from build123d import *

# Parameters (mm, degrees)
F0_W        = 100
F0_H        = 100
F1_DEPTH    = 50
F2_R        = 10
F3_T1_DEPTH = 150
F3_T4_ANGLE = 90
F3_T6_ANGLE = 90
F4_T1_DEPTH = 87.5
F4_T4_ANGLE = 90
F4_T6_ANGLE = 90
F5_R        = 30.8330010445
F6_DEPTH    = 40


# Not quite as in the source:
# - a fillet or chamfer that OpenCascade refuses, or shapes differently, is made with other operations: its cross-section is extruded or revolved along the edge and cut away or added


with BuildPart() as f1:
    # F0 (on Top) → F1 (new body)
    with BuildSketch(Plane.XY):
        with Locations((-16.9892802835, -14.8166164756)):
            Rectangle(F0_W, F0_H)
    extrude(amount=F1_DEPTH)

    # F2
    f2_edges = [f1.edges().sort_by_distance(p)[0] for p in [
        (-16.98928, -64.816616, 50),
        (33.01072, -14.816616, 50),
        (-16.98928, 35.183384, 50),
        (-66.98928, -14.816616, 50),
    ]]
    fillet(f2_edges, radius=F2_R)

    # F3: fillet of radius 40 on 2 edges, made by hand

    # F3_s2 → F3_t1 (cut)
    with BuildSketch(Plane.XY.offset(-100)):
        with BuildLine():
            ThreePointArc((33.0107197165, -24.8166164756), (21.294990964, -53.100887723), (-6.9892802835, -64.8166164756))
            Line((-6.9892802835, -64.8166164756), (33.0107197165, -64.8166164756))
            Line((33.0107197165, -64.8166164756), (33.0107197165, -24.8166164756))
        make_face()
        with BuildLine():
            ThreePointArc((-26.9892802835, 35.1833835244), (-55.2735515309, 23.4676547719), (-66.9892802835, -4.8166164756))
            Line((-66.9892802835, -4.8166164756), (-66.9892802835, 35.1833835244))
            Line((-66.9892802835, 35.1833835244), (-26.9892802835, 35.1833835244))
        make_face()
    extrude(amount=F3_T1_DEPTH, mode=Mode.SUBTRACT)

    # F3_s3 → F3_t4 (revolve, cut)
    with BuildSketch(Plane.YZ.offset(-26.9892802835)):
        with BuildLine():
            ThreePointArc((25.1833835244, 50), (32.2544513363, 47.0710678119), (35.1833835244, 40))
            Line((35.1833835244, 40), (35.1833835244, 50))
            Line((35.1833835244, 50), (25.1833835244, 50))
        make_face()
    revolve(axis=Axis((-26.9892802835, -4.8166164756, 50), (0, 0, 1)), revolution_arc=F3_T4_ANGLE, mode=Mode.SUBTRACT)

    # F3_s5 → F3_t6 (revolve, cut)
    with BuildSketch(Plane.YZ.offset(-6.9892802835)):
        with BuildLine():
            ThreePointArc((-54.8166164756, 50), (-61.8876842874, 47.0710678119), (-64.8166164756, 40))
            Line((-64.8166164756, 40), (-64.8166164756, 50))
            Line((-64.8166164756, 50), (-54.8166164756, 50))
        make_face()
    revolve(axis=Axis((-6.9892802835, -24.8166164756, 50), (0, 0, 1)), revolution_arc=F3_T6_ANGLE, mode=Mode.SUBTRACT)

    # F4: fillet of radius 15 on 2 edges, made by hand

    # F4_s2 → F4_t1 (cut)
    with BuildSketch(Plane.XY.offset(-37.5)):
        with BuildLine():
            ThreePointArc((33.0107197165, 20.1833835244), (28.6173214343, 30.7899852422), (18.0107197165, 35.1833835244))
            Line((18.0107197165, 35.1833835244), (33.0107197165, 35.1833835244))
            Line((33.0107197165, 35.1833835244), (33.0107197165, 20.1833835244))
        make_face()
        with BuildLine():
            ThreePointArc((-51.9892802835, -64.8166164756), (-62.5958820012, -60.4232181934), (-66.9892802835, -49.8166164756))
            Line((-66.9892802835, -49.8166164756), (-66.9892802835, -64.8166164756))
            Line((-66.9892802835, -64.8166164756), (-51.9892802835, -64.8166164756))
        make_face()
    extrude(amount=F4_T1_DEPTH, mode=Mode.SUBTRACT)

    # F4_s3 → F4_t4 (revolve, cut)
    with BuildSketch(Plane.XZ.offset(49.8166164756)):
        with BuildLine():
            ThreePointArc((-56.9892802835, 50), (-64.0603480953, 47.0710678119), (-66.9892802835, 40))
            Line((-66.9892802835, 40), (-66.9892802835, 50))
            Line((-66.9892802835, 50), (-56.9892802835, 50))
        make_face()
    revolve(axis=Axis((-51.9892802835, -49.8166164756, 50), (0, 0, 1)), revolution_arc=F4_T4_ANGLE, mode=Mode.SUBTRACT)

    # F4_s5 → F4_t6 (revolve, cut)
    with BuildSketch(Plane.XZ.offset(-20.1833835244)):
        with BuildLine():
            ThreePointArc((23.0107197165, 50), (30.0817875284, 47.0710678119), (33.0107197165, 40))
            Line((33.0107197165, 40), (33.0107197165, 50))
            Line((33.0107197165, 50), (23.0107197165, 50))
        make_face()
    revolve(axis=Axis((18.0107197165, 20.1833835244, 50), (0, 0, 1)), revolution_arc=F4_T6_ANGLE, mode=Mode.SUBTRACT)

    # F5 (on face) → F6 (cut)
    with BuildSketch(Plane.XY.offset(50)):
        with Locations((-16.8512575328, -14.6785899997)):
            Circle(F5_R)
    extrude(amount=-F6_DEPTH, mode=Mode.SUBTRACT)


solid = f1.part
Verification items for the finished model (mm, model axes). Round coordinates to 2 decimals unless told otherwise and drop trailing zeros. Loops run counter-clockwise (first coordinate to the right, second up) from the corner with the lowest first, then second, coordinate; pieces in that order, holes last. Notation, with made-up numbers: (-25, -40) - (-13, -40) arc R23 cw to (-13, -7) - close; hole circle Ø10 at (30, 53). An arc over 180 degrees is marked (long way). Answer in a Markdown table with one row per item. Add a question column.
Q1. Section check A-A on z = 25. Enter the section's corners in (x, y), plus the area to 3 significant figures.
Q2. Section check C-C on y = -21.5. Enter the section's corners in (x, z).
Q3. Section check B-B on z = 5. Enter the section's corners in (x, y).
Q4. Release check for a two-part mould opening along X. For faces 1 (the face through (-17, -14, 10)), 2 (the face through (-29.17, -61.97, 46.99)), 3 (the face through (12.56, -5.42, 30.28)), 4 (the face through (30.16, -2, 46.99)) record: pulls with the +X half, pulls with the -X half, needs draft (parallel to the pull), parting line crosses it, or undercut.
Q5. Gauge pin test, flat ends, axial feed: pin 1 (18.5 mm diameter, centred on x = -23.5, y = -30, fed in from +Z); pin 2 (1 mm diameter, centred on x = -28.5, z = 12, fed in from +Y); pin 3 (8 mm diameter, centred on y = -37, z = 11.5, fed in from +X). Record the tip position at first contact, or that the pin passes through.
Q6. Material ranges on line 1 (Z direction, x = 7, y = -26.5); line 2 (X direction, y = 6.5, z = 33.5); line 3 (X direction, y = 12.5, z = 38.5), recorded low to high.
Q7. Section check D-D on x = -15.5. Enter the section's corners in (y, z).
Found:
| question | item | result |
|---|---|---|
| 1 | outline | (-66.99, -49.82) arc R15 ccw to (-51.99, -64.82) - (-6.99, -64.82) arc R40 ccw to (33.01, -24.82) - (33.01, 20.18) arc R15 ccw to (18.01, 35.18) - (-26.99, 35.18) arc R40 ccw to (-66.99, -4.82) - close; hole circle Ø61.67 at (-16.85, -14.68) |
| 1 | area | 6,230 mm² |
| 2 | outline | (-66.99, 0) - (33.01, 0) - (33.01, 40) arc R10 ccw to (23.01, 50) - (13.22, 50) - (13.22, 10) - (-46.92, 10) - (-46.92, 50) - (-56.99, 50) arc R10 ccw to (-66.99, 40) - close |
| 3 | outline | (-66.99, -49.82) arc R15 ccw to (-51.99, -64.82) - (-6.99, -64.82) arc R40 ccw to (33.01, -24.82) - (33.01, 20.18) arc R15 ccw to (18.01, 35.18) - (-26.99, 35.18) arc R40 ccw to (-66.99, -4.82) - close |
| 4 | face 1 | undercut |
| 4 | face 2 | needs draft |
| 4 | face 3 | undercut |
| 4 | face 4 | pulls with the +X half |
| 5 | pin 1 | stops at z = 10 |
| 5 | pin 2 | stops at y = 35.17 |
| 5 | pin 3 | stops at x = 32.16 |
| 6 | line 1 | z = 0 to 10 |
| 6 | line 2 | x = -65.36 to -39.26, 5.56 to 33.01 |
| 6 | line 3 | x = -63.05 to -31.41, -2.29 to 33.01 |
| 7 | outline | (-64.82, 0) - (35.18, 0) - (35.18, 40) arc R10 ccw to (25.18, 50) - (16.12, 50) - (16.12, 10) - (-45.48, 10) - (-45.48, 50) - (-54.82, 50) arc R10 ccw to (-64.82, 40) - close |
